Design review of the part built by this model. Coordinates are the model's own, in mm. A direction names the side the tool comes from. Coordinates: 2 decimals unless noted, no trailing zeros. Loops run counter-clockwise (first coordinate to the right, second up) from the corner with the lowest first, then second, coordinate; pieces in that order, holes last.
Q1. Draft analysis for pull direction Z (two halves, no side actions). For faces 6 (the face through (-13.85, 8.62, -24.02)), 7 (the face through (-13.299, 1.109, 24.813)), 8 (the face through (-14.839, 1.109, -23.924)), 9 (the face through (-9, 114.3, 7)), state which applies: released by +Z, released by -Z, zero draft, split by the parting line, or undercut.
Q2. For P1, Ø15.5, axis at x = 27.5, y = 5.5, coming from the -Z side; P2, Ø10, axis at x = 9.5, y = 5.5, coming from the -Z side; P3, Ø24.5, axis at x = 30.5, y = -1, coming from the +Z side, all flat-tipped, find the tip position at first contact; note any pin that passes through.
Q3. Machinability: for faces 1 (the face through (-10.91, 31.31, -2.42)), 2 (the face through (28, 1, -0.889)), 3 (the face through (-10.91, 90.15, -2.42)), 4 (the face through (-14.066, -9.455, -24.388)), 5 (the face through (28, 1, 0.889)), which of the approach directions +Z, -Z, +X, -X, +Y, -Y give a long, thin tool a straight path to every point of the face, cutting with its end or side? Answer none if there is none.
Q4. Add section C-C on y = 69.5. Give the boundary of the cut face in (x, z).
Q5. Add section D-D on x = 32.5. Give the boundary of the cut face in (y, z), and give its area (3 significant figures).
Q6. Wall thickness on probe 1 along Z at (x, y) = (0, 24); probe 2 along X at (y, z) = (90, -5): over which ranges is each line inside the solid? List them lowest first.
Q7. Add section B-B on z = -2.5. Give the boundary of the cut face in (x, y) (1 decimal), and give its area (3 significant figures).
Q8. Add section A-A on x = 0. Give the boundary of the cut face in (y, z) (3 decimals), and give its area (3 significant figures).
```python
from build123d import *

# Parameters (mm, degrees)
SKETCH1_R           = 12.7
SKETCH1_R_2         = 11.176
BOSS_EXTRUDE1_DEPTH = 114.3
BOSS_EXTRUDE2_DEPTH = 0.889
CIRPATTERN1_COUNT   = 3
SKETCH3_R           = 11.176
SKETCH3_R_2         = 6.35
BOSS_EXTRUDE3_DEPTH = 3.175


with BuildPart() as part:
    # Sketch1 → Boss-Extrude1 (new body)
    with BuildSketch(Plane(origin=(0, 0, 0), x_dir=(1, 0, 0), z_dir=(0, 1, 0))):
        with Locations(Location((0, 0, 0), (0, 0, 270))):
            Circle(SKETCH1_R)
        with Locations(Location((0, 0, 0), (0, 0, 270))):
            Circle(SKETCH1_R_2, mode=Mode.SUBTRACT)
    extrude(amount=BOSS_EXTRUDE1_DEPTH)

    # Sketch2 → Boss-Extrude2 (add, symmetric)
    with BuildSketch(Plane.XY):
        Polygon((12.7, 0), (11.176, 0), (11.176, 20.32), (12.7, 20.32), (43.18, -3.408032613), (43.18, -18.648032613), align=None)
    boss_extrude2 = extrude(amount=BOSS_EXTRUDE2_DEPTH, both=True)

    # CirPattern1: Boss-Extrude2 ×3 about axis
    cirpattern1_axis = Axis((0, 0, 0), (0, 1, 0))
    for i in range(1, CIRPATTERN1_COUNT):
        add(boss_extrude2.rotate(cirpattern1_axis, i * 360 / CIRPATTERN1_COUNT))

    # Sketch3 → Boss-Extrude3 (add)
    with BuildSketch(Plane(origin=(0, 63.5, 0), x_dir=(1, 0, 0), z_dir=(0, 1, 0))):
        with Locations(Location((0, 0, 0), (0, 0, 270))):
            Circle(SKETCH3_R)
        with Locations(Location((0, 0, 0), (0, 0, 270))):
            Circle(SKETCH3_R_2, mode=Mode.SUBTRACT)
    extrude(amount=BOSS_EXTRUDE3_DEPTH)


solid = part.part
```
Entries:
1. face 6: released by -Z
1. face 7: released by +Z
1. face 8: undercut
1. face 9: zero draft
2. P1: stops at z = -0.89
2. P2: stops at z = -11.88
2. P3: stops at z = 0.89
3. face 1: -Y
3. face 2: -Z, +X, +Y, -Y
3. face 3: +Y
3. face 4: +X, -Y
3. face 5: +Z, +X, +Y, -Y
4. outline: circle Ø25.4 at (0, 0); hole circle Ø22.35 at (0, 0)
5. outline: (-12.11, -0.89) - (4.91, -0.89) - (4.91, 0.89) - (-12.11, 0.89) - close
5. area: 30.3 mm2
6. probe 1: z = -12.7 to -11.18, 11.18 to 12.7
6. probe 2: x = -11.67 to -10, 10 to 11.67
7. outline: (-12.5, 0) - (-10.9, 0) - (-10.9, 63.5) - (-5.8, 63.5) - (-5.8, 66.7) - (-10.9, 66.7) - (-10.9, 114.3) - (-12.5, 114.3) - close; (5.8, 63.5) - (10.9, 63.5) - (10.9, 0) - (12.5, 0) - (12.5, 114.3) - (10.9, 114.3) - (10.9, 66.7) - (5.8, 66.7) - close
7. area: 388 mm2
8. outline: (0, -12.7) - (114.3, -12.7) - (114.3, -11.176) - (66.675, -11.176) - (66.675, -6.35) - (63.5, -6.35) - (63.5, -11.176) - (0, -11.176) - close; (0, 11.176) - (63.5, 11.176) - (63.5, 6.35) - (66.675, 6.35) - (66.675, 11.176) - (114.3, 11.176) - (114.3, 12.7) - (0, 12.7) - close
8. area: 379 mm2
